Can you work these out from the drawing? Everything is in mm from the part's minimum corner. A direction names the side the tool comes from. Coordinates: 2 decimals unless noted, no trailing zeros. Order: outer loops, then holes, each group sorted by start corner. A loop starts at its lowest first (then second) coordinate and runs counter-clockwise, first axis right, second up. Notation, with made-up numbers: M 27,34.5 L 68,34.5 A23 cw 68,60.5 Z; hole C -9.75,54 d8. An arc over 180 degrees is marked long. Answer as a JSON object with one key per item and string values.
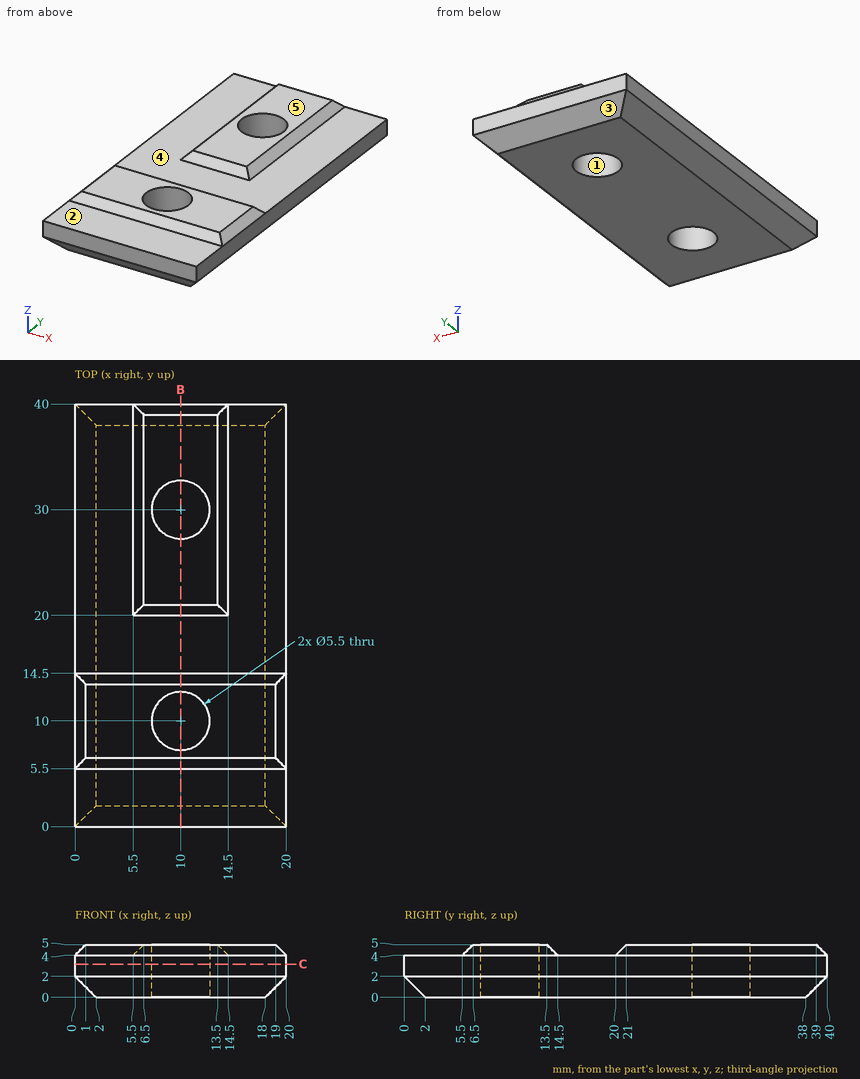
Item 1: I'm going to push flat-ended pins straight in: pin 1 (3 mm diameter, centred on x = 10, y = 1.5, fed in from +Z); pin 2 (2 mm diameter, centred on y = 15.5, z = 0.5, fed in from +X). Where does each tip first touch, or does it pass through?
Answers follow:
{"pin 1": "stops at z = 4", "pin 2": "stops at x = 19.5"}
Item 2: I want a section at B-B, the plane x = 10. Give the number of separate pieces and of enclosed holes in the cut face, plus the area to 3 significant figures.
Answers follow:
{"separate pieces": "3", "enclosed holes": "0", "area": "128 mm^2"}
Item 3: Which directions (+Z, -Z, +X, -X, +Y, -Y) give clear straight access to the entire face, cutting with the end or side of a thin tool? Please do the marked faces 1 and 2.
Answers follow:
{"face 1": "+Z, -Z", "face 2": "+Z, +X, -X, -Y"}
Item 4: I want a section at C-C, the plane z = 3.15. Write out the boundary of the cut face in (x, y), plus the area to 3 significant figures.
Answers follow:
{"outline": "M 0,0 L 20,0 L 20,40 L 0,40 Z; hole C 10,10 d5.5; hole C 10,30 d5.5", "area": "752 mm^2"}
Item 5: If we mould it in two halves opening along Y, with no side actions, what happens to the marked faces 3, 4 and 5? For each: pulls with the +Y half, pulls with the -Y half, needs draft (parallel to the pull), parting line crosses it, or undercut.
Answers follow:
{"face 3": "pulls with the +Y half", "face 4": "undercut", "face 5": "needs draft"}
Item 6: Please list where these lines run through material, in increasing order: line 1 (Y direction, x = 10, z = 3.5); line 2 (Y direction, x = 9.5, z = 0.4); line 3 (Y direction, x = 11.25, z = 4.3).
Answers follow:
{"line 1": "y = 0 to 7.25, 12.75 to 27.25, 32.75 to 40", "line 2": "y = 1.6 to 7.3, 12.7 to 27.3, 32.7 to 38.4", "line 3": "y = 5.8 to 7.55, 12.45 to 14.2, 20.3 to 27.55, 32.45 to 39.7"}
